Drawing for the job (mm, zero at the part's lowest x, y, z). A direction names the side the tool comes from. Coordinates: 2 decimals unless noted, no trailing zeros. Order: outer loops, then holes, each group sorted by start corner. A loop starts at its lowest first (then second) coordinate and runs counter-clockwise, first axis right, second up.
1) Cut at A-A (y = 45). List the corners of the cut face in (x, z), and give its area (3 significant figures).
2) Mould opens along Z. For the marked faces 1, 2, 3 and 4 say: +Z half, -Z half, draft (parallel to the pull), parting line (faces both ways), or undercut.
3) Cut at B-B (z = 10). List the corners of the cut face in (x, y), and give its area (3 significant figures).
4) Cut at D-D (z = 16.25). List the corners of the cut face in (x, y), and give its area (3 significant figures).
5) Cut at C-C (x = 70). List the corners of the cut face in (y, z).
6) Tool access for the marked faces 5 and 6: list every direction of +Z, -Z, +X, -X, +Y, -Y with a clear straight run to the whole face (end or side of a thin tool).
7) Wall check: L1, parallel to X at y = 19, z = 10; L2, parallel to X at y = 34, z = 8.75; L3, parallel to X at y = 46, z = 10. Give the ranges that are in metal, low to high.
8) Pin check, flat tips, straight feed: pin 1 Ø8 at (x, z) = (65.5, 11.5) entering from -Y; pin 2 Ø12 at (x, z) = (70, 10) entering from +Y; pin 3 Ø5 at (y, z) = (60.5, 10) entering from +X. Stop position of each tip, or through.
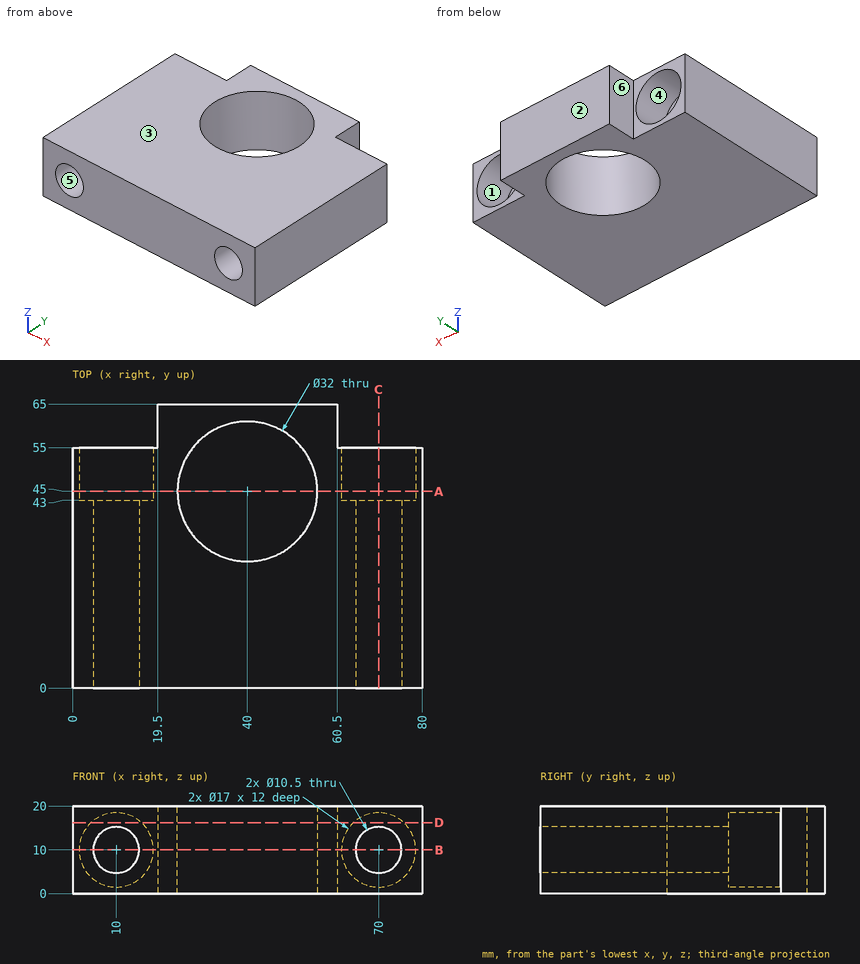
Geometry check:
1. outline: (0, 0) - (24, 0) - (24, 20) - (0, 20) - close; (56, 0) - (80, 0) - (80, 20) - (56, 20) - close; hole circle Ø17 at (10, 10); hole circle Ø17 at (70, 10)
1. area: 506 mm2
2. face 1: undercut
2. face 2: draft
2. face 3: +Z half
2. face 4: undercut
3. outline: (0, 0) - (4.75, 0) - (4.75, 43) - (1.5, 43) - (1.5, 55) - (0, 55) - close; (15.25, 0) - (64.75, 0) - (64.75, 43) - (61.5, 43) - (61.5, 55) - (60.5, 55) - (60.5, 65) - (19.5, 65) - (19.5, 55) - (18.5, 55) - (18.5, 43) - (15.25, 43) - close; (75.25, 0) - (80, 0) - (80, 55) - (78.5, 55) - (78.5, 43) - (75.25, 43) - close; hole circle Ø32 at (40, 45)
3. area: 2,690 mm2
4. outline: (0, 0) - (80, 0) - (80, 55) - (75.76, 55) - (75.76, 43) - (64.24, 43) - (64.24, 55) - (60.5, 55) - (60.5, 65) - (19.5, 65) - (19.5, 55) - (15.76, 55) - (15.76, 43) - (4.24, 43) - (4.24, 55) - (0, 55) - close; hole circle Ø32 at (40, 45)
4. area: 3,730 mm2
5. outline: (0, 0) - (55, 0) - (55, 1.5) - (43, 1.5) - (43, 4.75) - (0, 4.75) - close; (0, 15.25) - (43, 15.25) - (43, 18.5) - (55, 18.5) - (55, 20) - (0, 20) - close
6. face 5: +Y, -Y
6. face 6: +Z, -Z, -X, +Y
7. L1: x = 0 to 4.75, 15.25 to 64.75, 75.25 to 80
7. L2: x = 0 to 4.9, 15.1 to 28.38, 51.62 to 64.9, 75.1 to 80
7. L3: x = 0 to 1.5, 18.5 to 24.03, 55.97 to 61.5, 78.5 to 80
8. pin 1: stops at y = 0
8. pin 2: stops at y = 43
8. pin 3: stops at x = 60.5
